```python
from build123d import *

# Parameters (mm, degrees)
CUT_EXTRUDE_2_DEPTH      = 0.12
CUT_EXTRUDE_2_DEPTH_BACK = 0.12
CUT_EXTRUDE_3_DEPTH      = 0.12
CUT_EXTRUDE_3_DEPTH_BACK = 0.12


with BuildPart() as part:
    # Sketch 1 → Revolve 1 (revolve)
    with BuildSketch(Plane.XY):
        with BuildLine():
            Line((0, 0), (-0.5, 0))
            Line((-0.5, 0), (-0.8, 0.3))
            Line((-0.8, 0.3), (-0.8, 13.04))
            ThreePointArc((-0.8, 13.04), (-0.830448187, 13.193073373), (-0.917157288, 13.322842712))
            Line((-0.917157288, 13.322842712), (-1.5, 13.905685425))
            Line((-1.5, 13.905685425), (-1.5, 14))
            Line((-1.5, 14), (-0.4, 14))
            Line((-0.4, 14), (-0.320283434, 12.86))
            Line((-0.320283434, 12.86), (0, 12.86))
            Line((0, 12.86), (0, 0))
        make_face()
    revolve(axis=Axis((0, 12.86, 0), (0, -1, 0)))

    # Sketch 3 → Cut-Extrude 2 (cut, two sides)
    with BuildSketch(Plane.XY) as cut_extrude_2_sk:
        Polygon((-0.9, 14), (-0.343984849, 12.86), (0.343984849, 12.86), (0.9, 14), align=None)
    extrude(amount=CUT_EXTRUDE_2_DEPTH, mode=Mode.SUBTRACT)
    extrude(cut_extrude_2_sk.sketch, amount=-CUT_EXTRUDE_2_DEPTH_BACK, mode=Mode.SUBTRACT)

    # Sketch 4 → Cut-Extrude 3 (cut, two sides)
    with BuildSketch(Plane(origin=(0, 0, 0), x_dir=(0, 0, -1), z_dir=(1, 0, 0))) as cut_extrude_3_sk:
        Polygon((-0.343984849, 12.86), (-0.9, 14), (0.9, 14), (0.343984849, 12.86), align=None)
    extrude(amount=CUT_EXTRUDE_3_DEPTH, mode=Mode.SUBTRACT)
    extrude(cut_extrude_3_sk.sketch, amount=-CUT_EXTRUDE_3_DEPTH_BACK, mode=Mode.SUBTRACT)


solid = part.part
```
The listing builds one solid part. Answer for the finished solid, in the listing's coordinates (mm). A direction names the side the tool comes from. Round coordinates to 2 decimals unless told otherwise and drop trailing zeros. Order: outer loops, then holes, each group sorted by start corner. A loop starts at its lowest first (then second) coordinate and runs counter-clockwise, first axis right, second up. Notation, with made-up numbers: (-19, 31.25) - (6, 31.25) arc R14 cw to (6, 36.25) - close; hole circle Ø8 at (48, 58.5). An arc over 180 degrees is marked (long way). Put each result on its own line as item: value. Start each with the question number.
(1) Find section C-C (y = 7.5). Give the vertices of the cut face in (x, z).
(2) Find section B-B (x = 0). Give the vertices of the cut face in (y, z).
(3) Straight lines are drawn through the part: probe 1 along Z at (x, y) = (0.35, 8.5); probe 2 along Y at (x, z) = (0.95, 0.15); probe 3 along Z at (x, y) = (-0.1, 7.5). For each, find the intervals that lie inside material, in ascending order. Write a range as from..to.
(4) Given P1, Ø1.5, axis at y = 6.5, z = 0.5, coming from the -X side; P2, Ø1, axis at x = -0.5, y = 12, coming from the -Z side; P3, Ø0.7, axis at y = 13.5, z = 0.5, coming from the +X side, each flat-ended and moving along its own axis, determine where each tip first touches the part or whether it passes through.
(5) For faces 1 (the flat face through (0.4, 14, -0.4)), 2 (the cylindrical face through (0.63, 6.76, 0.49)), determine the directions among +Z, -Z, +X, -X, +Y, -Y from which every point of the face is accessible in a straight line to the end or side of a thin tool.
(6) Find section A-A (z = 0). Give the vertices of the cut face in (x, y).
Reply:
1. outline: circle Ø1.6 at (0, 0)
2. outline: (0, -0.5) - (0.3, -0.8) - (13.04, -0.8) arc R0.4 cw to (13.32, -0.92) - (13.91, -1.5) - (14, -1.5) - (14, -0.9) - (12.86, -0.34) - (12.86, 0.34) - (14, 0.9) - (14, 1.5) - (13.91, 1.5) - (13.32, 0.92) arc R0.4 cw to (13.04, 0.8) - (0.3, 0.8) - (0, 0.5) - close
3. probe 1: -0.72..0.72
3. probe 2: 13.37..14
3. probe 3: -0.79..0.79
4. P1: x = -0.8
4. P2: z = -0.8
4. P3: x = 1.37
5. face 1: +Z, -Z, +X, -X, +Y
5. face 2: -Y
6. outline: (-1.5, 13.91) - (-0.92, 13.32) arc R0.4 cw to (-0.8, 13.04) - (-0.8, 0.3) - (-0.5, 0) - (0.5, 0) - (0.8, 0.3) - (0.8, 13.04) arc R0.4 cw to (0.92, 13.32) - (1.5, 13.91) - (1.5, 14) - (0.9, 14) - (0.34, 12.86) - (-0.34, 12.86) - (-0.9, 14) - (-1.5, 14) - close
